```python
from build123d import *

# Parameters (mm, degrees)
SKETCH1_R              = 16.05
SKETCH1_R_2            = 1.65
BASE_DEPTH             = 3.175
SKETCH3_R              = 1.65
STRUT_HOLES_DEPTH      = 4.175
LIGHTENING_HOLES_DEPTH = 4.175


with BuildPart() as part:
    # Sketch1 → Base (new body)
    with BuildSketch(Plane.XY):
        with BuildLine():
            Line((-113.35576806, -30.824729171), (-235.437134887, -94.376266227))
            ThreePointArc((-235.437134887, -94.376266227), (-237.896976574, -97.307791395), (-237.563445987, -101.120063459))
            Line((-237.563445987, -101.120063459), (-219.093501457, -136.600496786))
            ThreePointArc((-219.093501457, -136.600496786), (-216.161976289, -139.060338474), (-212.349704225, -138.726807886))
            Line((-212.349704225, -138.726807886), (-101.120845899, -80.824729171))
            ThreePointArc((-101.120845899, -80.824729171), (-95.519277876, -78.716448255), (-89.577130568, -78))
            Line((-89.577130568, -78), (89.577130568, -78))
            ThreePointArc((89.577130568, -78), (95.519277876, -78.716448255), (101.120845899, -80.824729171))
            Line((101.120845899, -80.824729171), (212.349704225, -138.726807886))
            ThreePointArc((212.349704225, -138.726807886), (216.161976289, -139.060338474), (219.093501457, -136.600496786))
            Line((219.093501457, -136.600496786), (237.563445987, -101.120063459))
            ThreePointArc((237.563445987, -101.120063459), (237.896976574, -97.307791395), (235.437134887, -94.376266227))
            Line((235.437134887, -94.376266227), (113.35576806, -30.824729171))
            ThreePointArc((113.35576806, -30.824729171), (107.754200038, -28.716448255), (101.812052729, -28))
            Line((101.812052729, -28), (-101.812052729, -28))
            ThreePointArc((-101.812052729, -28), (-107.754200038, -28.716448255), (-113.35576806, -30.824729171))
        make_face()
        with Locations((-200, -104.11341011)):
            Circle(SKETCH1_R, mode=Mode.SUBTRACT)
        with Locations((-221.458631392, -97.347529622)):
            Circle(SKETCH1_R_2, mode=Mode.SUBTRACT)
        with Locations((-193.234119511, -82.654778719)):
            Circle(SKETCH1_R_2, mode=Mode.SUBTRACT)
        with Locations((-178.541368608, -110.879290599)):
            Circle(SKETCH1_R_2, mode=Mode.SUBTRACT)
        with Locations((-206.765880489, -125.572041502)):
            Circle(SKETCH1_R_2, mode=Mode.SUBTRACT)
        with Locations((206.765880489, -125.572041502)):
            Circle(SKETCH1_R_2, mode=Mode.SUBTRACT)
        with Locations((221.458631392, -97.347529622)):
            Circle(SKETCH1_R_2, mode=Mode.SUBTRACT)
        with Locations((193.234119511, -82.654778719)):
            Circle(SKETCH1_R_2, mode=Mode.SUBTRACT)
        with Locations((178.541368608, -110.879290599)):
            Circle(SKETCH1_R_2, mode=Mode.SUBTRACT)
        with Locations((200, -104.11341011)):
            Circle(SKETCH1_R, mode=Mode.SUBTRACT)
        with Locations((-10, -47.226497308)):
            Circle(SKETCH1_R_2, mode=Mode.SUBTRACT)
        with Locations((10, -47.226497308)):
            Circle(SKETCH1_R_2, mode=Mode.SUBTRACT)
        with Locations((0, -64.547005384)):
            Circle(SKETCH1_R_2, mode=Mode.SUBTRACT)
    extrude(amount=BASE_DEPTH)

    # Sketch3 → Strut Holes (cut, through all)
    with BuildSketch(Plane.XY.offset(3.175)):
        with Locations((-214.658447291, -134.29175372)):
            Circle(SKETCH3_R)
        with Locations((-148.132634803, -99.660607727)):
            Circle(SKETCH3_R)
        with Locations((-78.03119405, -73)):
            Circle(SKETCH3_R)
        with Locations((-78.03119405, -33)):
            Circle(SKETCH3_R)
        with Locations((-166.602579332, -64.1801744)):
            Circle(SKETCH3_R)
        with Locations((-233.128391821, -98.811320393)):
            Circle(SKETCH3_R)
        with Locations((233.128391821, -98.811320393)):
            Circle(SKETCH3_R)
        with Locations((166.602579332, -64.1801744)):
            Circle(SKETCH3_R)
        with Locations((78.03119405, -33)):
            Circle(SKETCH3_R)
        with Locations((78.03119405, -73)):
            Circle(SKETCH3_R)
        with Locations((148.132634803, -99.660607727)):
            Circle(SKETCH3_R)
        with Locations((214.658447291, -134.29175372)):
            Circle(SKETCH3_R)
    extrude(amount=-STRUT_HOLES_DEPTH, mode=Mode.SUBTRACT)

    # Sketch4 → Lightening Holes (cut, through all)
    with BuildSketch(Plane(origin=(0, 0, 0), x_dir=(-1, 0, 0), z_dir=(0, 0, -1))):
        with BuildLine():
            Line((-166.732564066, -103.70620831), (-160.358460468, -100.38806))
            ThreePointArc((-160.358460468, -100.38806), (-158.749015825, -99.059097441), (-157.82234729, -97.188873132))
            ThreePointArc((-157.82234729, -97.188873132), (-152.750120935, -90.790499395), (-144.599570492, -90.305531214))
            ThreePointArc((-144.599570492, -90.305531214), (-142.53605719, -90.619165384), (-140.52429527, -90.063047123))
            Line((-140.52429527, -90.063047123), (-105.738332031, -71.954620839))
            ThreePointArc((-105.738332031, -71.954620839), (-98.269905543, -69.096671797), (-90.347714306, -68.008483875))
            ThreePointArc((-90.347714306, -68.008483875), (-88.493641512, -67.607748759), (-86.922263791, -66.545229763))
            Line((-86.922263791, -66.545229763), (-79.009491694, -58.632457666))
            ThreePointArc((-79.009491694, -58.632457666), (-77.556385787, -54.760066484), (-79.516892411, -51.11817906))
            Line((-79.516892411, -51.11817906), (-92.727653164, -41.063765898))
            ThreePointArc((-92.727653164, -41.063765898), (-100.534196684, -38.054529652), (-108.738281928, -39.694837502))
            Line((-108.738281928, -39.694837502), (-154.376753667, -63.452722127))
            ThreePointArc((-154.376753667, -63.452722127), (-155.986198311, -64.781684686), (-156.912866845, -66.651908996))
            ThreePointArc((-156.912866845, -66.651908996), (-161.9850932, -73.050282732), (-170.135643643, -73.535250914))
            ThreePointArc((-170.135643643, -73.535250914), (-172.199156946, -73.221616743), (-174.210918865, -73.777735004))
            Line((-174.210918865, -73.777735004), (-180.585022463, -77.095883315))
            ThreePointArc((-180.585022463, -77.095883315), (-182.645072259, -79.099137955), (-183.262226102, -81.905551227))
            ThreePointArc((-183.262226102, -81.905551227), (-183.239750678, -82.990325484), (-183.334932996, -84.071149549))
            ThreePointArc((-183.334932996, -84.071149549), (-183.171057415, -86.227404823), (-182.1120053, -88.112796196))
            ThreePointArc((-182.1120053, -88.112796196), (-178.711740004, -93.031443393), (-176.632932149, -98.637997792))
            ThreePointArc((-176.632932149, -98.637997792), (-175.695957289, -100.586938562), (-174.023651545, -101.957954795))
            ThreePointArc((-174.023651545, -101.957954795), (-173.083697968, -102.499921221), (-172.207994291, -103.140532962))
            ThreePointArc((-172.207994291, -103.140532962), (-169.555130221, -104.244682653), (-166.732564066, -103.70620831))
        make_face()
        with BuildLine():
            Line((-68.284399705, -68), (-63.199367137, -68))
            ThreePointArc((-63.199367137, -68), (-61.351608072, -66.765366865), (-61.785153575, -64.585786438))
            Line((-61.785153575, -64.585786438), (-68.424239552, -57.946700461))
            ThreePointArc((-68.424239552, -57.946700461), (-69.838453114, -57.360914023), (-71.252666676, -57.946700461))
            Line((-71.252666676, -57.946700461), (-74.132142401, -60.826176185))
            ThreePointArc((-74.132142401, -60.826176185), (-74.691303243, -62.565648815), (-73.60347304, -64.033658123))
            ThreePointArc((-73.60347304, -64.033658123), (-71.563592326, -65.373065627), (-69.908865429, -67.166666667))
            ThreePointArc((-69.908865429, -67.166666667), (-69.197270634, -67.779513042), (-68.284399705, -68))
        make_face()
        with BuildLine():
            Line((-25.430550415, -40.5), (-13.883545032, -60.5))
            ThreePointArc((-13.883545032, -60.5), (-13.883545032, -65.5), (-18.21367205, -68))
            Line((-18.21367205, -68), (-49.228804389, -68))
            ThreePointArc((-49.228804389, -68), (-51.14222155, -67.619397663), (-52.764338294, -66.535533906))
            Line((-52.764338294, -66.535533906), (-72.764338294, -46.535533906))
            ThreePointArc((-72.764338294, -46.535533906), (-73.848202051, -41.086582838), (-69.228804389, -38))
            Line((-69.228804389, -38), (-29.760677434, -38))
            ThreePointArc((-29.760677434, -38), (-27.260677434, -38.669872981), (-25.430550415, -40.5))
        make_face()
        with BuildLine():
            Line((52.764338294, -66.535533906), (72.764338294, -46.535533906))
            ThreePointArc((72.764338294, -46.535533906), (73.848202051, -41.086582838), (69.228804389, -38))
            Line((69.228804389, -38), (29.760677434, -38))
            ThreePointArc((29.760677434, -38), (27.260677434, -38.669872981), (25.430550415, -40.5))
            Line((25.430550415, -40.5), (13.883545032, -60.5))
            ThreePointArc((13.883545032, -60.5), (13.883545032, -65.5), (18.21367205, -68))
            Line((18.21367205, -68), (49.228804389, -68))
            ThreePointArc((49.228804389, -68), (51.14222155, -67.619397663), (52.764338294, -66.535533906))
        make_face()
        with BuildLine():
            Line((68.284399705, -68), (63.199367137, -68))
            ThreePointArc((63.199367137, -68), (61.351608072, -66.765366865), (61.785153575, -64.585786438))
            Line((61.785153575, -64.585786438), (68.424239552, -57.946700461))
            ThreePointArc((68.424239552, -57.946700461), (69.838453114, -57.360914023), (71.252666676, -57.946700461))
            Line((71.252666676, -57.946700461), (74.132142401, -60.826176185))
            ThreePointArc((74.132142401, -60.826176185), (74.691303243, -62.565648815), (73.60347304, -64.033658123))
            ThreePointArc((73.60347304, -64.033658123), (71.563592326, -65.373065627), (69.908865429, -67.166666667))
            ThreePointArc((69.908865429, -67.166666667), (69.197270634, -67.779513042), (68.284399705, -68))
        make_face()
        with BuildLine():
            Line((154.376753667, -63.452722127), (108.738281928, -39.694837502))
            ThreePointArc((108.738281928, -39.694837502), (100.534196684, -38.054529652), (92.727653164, -41.063765898))
            Line((92.727653164, -41.063765898), (79.516892411, -51.11817906))
            ThreePointArc((79.516892411, -51.11817906), (77.556385787, -54.760066484), (79.009491694, -58.632457666))
            Line((79.009491694, -58.632457666), (86.922263791, -66.545229763))
            ThreePointArc((86.922263791, -66.545229763), (88.493641512, -67.607748759), (90.347714306, -68.008483875))
            ThreePointArc((90.347714306, -68.008483875), (98.269905543, -69.096671797), (105.738332031, -71.954620839))
            Line((105.738332031, -71.954620839), (140.52429527, -90.063047123))
            ThreePointArc((140.52429527, -90.063047123), (142.53605719, -90.619165384), (144.599570492, -90.305531214))
            ThreePointArc((144.599570492, -90.305531214), (152.750120935, -90.790499395), (157.82234729, -97.188873132))
            ThreePointArc((157.82234729, -97.188873132), (158.749015825, -99.059097441), (160.358460468, -100.38806))
            Line((160.358460468, -100.38806), (166.732564066, -103.70620831))
            ThreePointArc((166.732564066, -103.70620831), (169.555130221, -104.244682653), (172.207994291, -103.140532962))
            ThreePointArc((172.207994291, -103.140532962), (173.083697968, -102.499921221), (174.023651545, -101.957954795))
            ThreePointArc((174.023651545, -101.957954795), (175.695957289, -100.586938562), (176.632932149, -98.637997792))
            ThreePointArc((176.632932149, -98.637997792), (178.711740004, -93.031443393), (182.1120053, -88.112796196))
            ThreePointArc((182.1120053, -88.112796196), (183.171057415, -86.227404823), (183.334932996, -84.071149549))
            ThreePointArc((183.334932996, -84.071149549), (183.239750678, -82.990325484), (183.262226102, -81.905551227))
            ThreePointArc((183.262226102, -81.905551227), (182.645072259, -79.099137955), (180.585022463, -77.095883315))
            Line((180.585022463, -77.095883315), (174.210918865, -73.777735004))
            ThreePointArc((174.210918865, -73.777735004), (172.199156946, -73.221616743), (170.135643643, -73.535250914))
            ThreePointArc((170.135643643, -73.535250914), (161.9850932, -73.050282732), (156.912866845, -66.651908996))
            ThreePointArc((156.912866845, -66.651908996), (155.986198311, -64.781684686), (154.376753667, -63.452722127))
        make_face()
    extrude(amount=-LIGHTENING_HOLES_DEPTH, mode=Mode.SUBTRACT)


solid = part.part
```
Design review of the part built by this model. Coordinates are the model's own, in mm. A direction names the side the tool comes from. Give positions to 0.01 mm unless a question says otherwise; leave off trailing zeros. Order: outer loops, then holes, each group sorted by start corner. A loop starts at its lowest first (then second) coordinate and runs counter-clockwise, first axis right, second up. Notation, with made-up numbers: (21.25, 82) - (75.25, 82) arc R18 cw to (75.25, 93) - close; hole circle Ø7 at (-26.75, 40.25). An arc over 180 degrees is marked (long way). Use a Markdown table: item, result. Add a question column.
(1) Mouldability with a two-part tool opening along Y and no side actions: class faces 3 (the face through (-173.542, -62.156, 1.565)), 4 (the face through (123.375, -81.136, 1.565)), 5 (the face through (-122.888, -80.882, 1.565)), 6 (the face through (155.96, -109.37, 1.57)) as +Y half, -Y half, draft (parallel to the pull), parting line (faces both ways), or undercut.
(2) Add section A-A on x = 135.5. Give the boundary of the cut face in (y, z) (3 decimals).
(3) Clearance check with flat-ended pins moving along their axes: P1, Ø1.5, axis at x = -101.5, z = 0.5, coming from the -Y side; P2, Ø12, axis at x = 52.5, y = -78.5, coming from the +Z side (3 decimals). State where each tip first meets the part, or that it passes through.
(4) Add section B-B on z = 2.2. Give the number of separate pieces and of enclosed holes in the cut face, then the cut area to 3 significant figures.
(5) Add section C-C on x = 200. Give the boundary of the cut face in (y, z) (3 decimals), then the cut area to 3 significant figures.
(6) Machinability: for faces 1 (the face through (-228.46, -118.61, 1.57)), 2 (the face through (-86.215, -46.021, 1.565)), which of the approach directions +Z, -Z, +X, -X, +Y, -Y give a long, thin tool a straight path to every point of the face, cutting with its end or side? Answer none if there is none.
(7) Wall thickness on probe 1 along Y at (x, z) = (32.5, 1); probe 2 along Y at (x, z) = (-214.5, 1.8); probe 3 along Y at (x, z) = (-193.5, 2.7): over which ranges is each line inside the solid? List them lowest first. Write a range as [from, to].
Report:
| question | item | result |
|---|---|---|
| 1 | face 3 | +Y half |
| 1 | face 4 | undercut |
| 1 | face 5 | undercut |
| 1 | face 6 | -Y half |
| 2 | outline | (-98.721, 0) - (-87.448, 0) - (-87.448, 3.175) - (-98.721, 3.175) - close; (-53.626, 0) - (-42.352, 0) - (-42.352, 3.175) - (-53.626, 3.175) - close |
| 3 | P1 | stops at y = -81.41 |
| 3 | P2 | stops at z = 3.175 |
| 4 | separate pieces | 1 |
| 4 | enclosed holes | 31 |
| 4 | area | 13,700 mm² |
| 5 | outline | (-132.298, 0) - (-120.163, 0) - (-120.163, 3.175) - (-132.298, 3.175) - close; (-88.063, 0) - (-75.929, 0) - (-75.929, 3.175) - (-88.063, 3.175) - close |
| 5 | area | 77.1 mm² |
| 6 | face 1 | +Z, -Z, -X, -Y |
| 6 | face 2 | +Z, -Z |
| 7 | probe 1 | y = [-78, -68], [-38, -28] |
| 7 | probe 2 | y = [-139.29, -135.93], [-132.65, -110.99], [-97.23, -83.48] |
| 7 | probe 3 | y = [-128.91, -118.79], [-89.44, -84.28], [-81.03, -72.55] |
